```python
from build123d import *

# Parameters (mm, degrees)
EXTRUDE_1_DEPTH     = 20
CUT_EXTRUDE_1_REACH = 47.924
SKETCH_2_R          = 4
CUT_EXTRUDE_2_REACH = 47.924
SKETCH_3_R          = 1.5


with BuildPart() as part:
    # 草图1 → 凸台-拉伸1 (new body)
    with BuildSketch(Plane(origin=(0, 0, 0), x_dir=(0, 0, -1), z_dir=(1, 0, 0))):
        Polygon((0, 0), (0, 22), (3, 22), (3, -3), (-35, -3), (-35, 0), align=None)
    extrude(amount=EXTRUDE_1_DEPTH)

    # 草图2 → 切除-拉伸1 (cut, up to next)
    with BuildSketch(Plane.XY, mode=Mode.PRIVATE) as cut_extrude_1_sk1:
        with Locations((10, 13)):
            Circle(SKETCH_2_R)
    cut_extrude_1_tool1 = extrude(cut_extrude_1_sk1.sketch, amount=-CUT_EXTRUDE_1_REACH, mode=Mode.PRIVATE) & part.part
    add(cut_extrude_1_tool1.solids().sort_by_distance((10, 13, 0))[0], mode=Mode.SUBTRACT)

    # 草图3 → 切除-拉伸2 (cut, up to next)
    with BuildSketch(Plane(origin=(0, 0, 0), x_dir=(1, 0, 0), z_dir=(0, 1, 0)), mode=Mode.PRIVATE) as cut_extrude_2_sk1:
        with Locations(Location((4, -6, 0), (0, 0, 270))):
            Circle(SKETCH_3_R)
    cut_extrude_2_tool1 = extrude(cut_extrude_2_sk1.sketch, amount=-CUT_EXTRUDE_2_REACH, mode=Mode.PRIVATE) & part.part
    # 草图3 → 切除-拉伸2 (cut, up to next)
    with BuildSketch(Plane(origin=(0, 0, 0), x_dir=(1, 0, 0), z_dir=(0, 1, 0)), mode=Mode.PRIVATE) as cut_extrude_2_sk2:
        with Locations(Location((16, -6, 0), (0, 0, 270))):
            Circle(SKETCH_3_R)
    cut_extrude_2_tool2 = extrude(cut_extrude_2_sk2.sketch, amount=-CUT_EXTRUDE_2_REACH, mode=Mode.PRIVATE) & part.part
    add(cut_extrude_2_tool1.solids().sort_by_distance((4, 0, 6))[0], mode=Mode.SUBTRACT)
    add(cut_extrude_2_tool2.solids().sort_by_distance((16, 0, 6))[0], mode=Mode.SUBTRACT)


solid = part.part
```
Part model, mm, in its own coordinate system. A direction names the side the tool comes from. Round coordinates to 2 decimals unless told otherwise and drop trailing zeros. Loops run counter-clockwise (first coordinate to the right, second up) from the corner with the lowest first, then second, coordinate; pieces in that order, holes last. Notation, with made-up numbers: (-21.5, -4.5) -> (27.5, -4.5) arc R10 ccw to (27.5, 0.5) -> close; hole circle Ø8 at (60.5, 41.25). An arc over 180 degrees is marked (long way). Use a Markdown table: item, result.
1) Drop flat-ended pins along their axis: pin 1 Ø2.5 at (x, z) = (16, 6) entering from -Y; pin 2 Ø6 at (x, y) = (12, 16.5) entering from +Z; pin 3 Ø10 at (y, z) = (2.5, 29.5) entering from -X. Give the stop position or say it passes through.
The answers:
| item | result |
|---|---|
| pin 1 | passes through |
| pin 2 | stops at z = 0 |
| pin 3 | stops at x = 0 |
2) Cut at C-C, the plane y = 13. List the corners of the cut face in (x, z), and give its area (3 significant figures).
The answers:
| item | result |
|---|---|
| outline | (0, -3) -> (6, -3) -> (6, 0) -> (0, 0) -> close; (14, -3) -> (20, -3) -> (20, 0) -> (14, 0) -> close |
| area | 36.0 mm2 |
3) Pull direction Y, two halves, no side cores. Call faces 3 (the flat face through (0, -1, 9)), 4 (the cylindrical face through (7.05, 15.7, -1.48)), 5 (the flat face through (10, -3, 16)): pulls with the +Y half, pulls with the -Y half, needs draft (parallel to the pull), parting line crosses it, or undercut.
The answers:
| item | result |
|---|---|
| face 3 | needs draft |
| face 4 | undercut |
| face 5 | pulls with the -Y half |
4) Probe line 1 (X direction, y = -1.05, z = 6); line 2 (Y direction, x = 10, z = -0.85); line 3 (Z direction, x = 15.25, y = 11.25). List the from-to ranges inside material, lowest first. Write a range as [from, to].
The answers:
| item | result |
|---|---|
| line 1 | x = [0, 2.5], [5.5, 14.5], [17.5, 20] |
| line 2 | y = [-3, 9], [17, 22] |
| line 3 | z = [-3, 0] |
5) Cut at A-A, the plane x = 4. List the corners of the cut face in (y, z).
The answers:
| item | result |
|---|---|
| outline | (-3, -3) -> (22, -3) -> (22, 0) -> (0, 0) -> (0, 4.5) -> (-3, 4.5) -> close; (-3, 7.5) -> (0, 7.5) -> (0, 35) -> (-3, 35) -> close |
6) Tool access for faces 1 (the flat face through (10, 0, 18)), 2 (the cylindrical face through (17.01, -1.48, 4.89)): list every direction of +Z, -Z, +X, -X, +Y, -Y with a clear straight run to the whole face (end or side of a thin tool).
The answers:
| item | result |
|---|---|
| face 1 | +Z, +X, -X, +Y |
| face 2 | +Y, -Y |
7) Cut at B-B, the plane z = 6. List the corners of the cut face in (x, y), and give its area (3 significant figures).
The answers:
| item | result |
|---|---|
| outline | (0, -3) -> (2.5, -3) -> (2.5, 0) -> (0, 0) -> close; (5.5, -3) -> (14.5, -3) -> (14.5, 0) -> (5.5, 0) -> close; (17.5, -3) -> (20, -3) -> (20, 0) -> (17.5, 0) -> close |
| area | 42.0 mm2 |
8) Cut at D-D, the plane y = -0.5. List the corners of the cut face in (x, z), and give its area (3 significant figures).
The answers:
| item | result |
|---|---|
| outline | (0, -3) -> (20, -3) -> (20, 35) -> (0, 35) -> close; hole circle Ø3 at (4, 6); hole circle Ø3 at (16, 6) |
| area | 746 mm2 |
